```python
from build123d import *

# Parameters (mm, degrees)
BOSS_EXTRUDE1_DEPTH = 146.05
BOSS_EXTRUDE2_DEPTH = 6.35
SKETCH3_W           = 274.391313821
SKETCH3_H           = 212.158232336
CUT_EXTRUDE1_DEPTH  = 81.28
SKETCH4_W           = 56.814403599
SKETCH4_H           = 146.05
SKETCH4_W_2         = 112.041307198
CUT_EXTRUDE2_DEPTH  = 269.802733384


with BuildPart() as part:
    # Sketch1 → Boss-Extrude1 (new body)
    with BuildSketch(Plane.XY):
        Polygon((0, 0), (0, 107.95), (3.175, 107.95), (7.6109518, 6.35), (50.7909518, 6.35), (55.226903599, 107.95), (58.401903599, 107.95), (62.837855399, 6.35), (106.017855399, 6.35), (110.453807198, 107.95), (113.628807198, 107.95), (118.064758998, 6.35), (161.244758998, 6.35), (165.680710797, 107.95), (168.855710797, 107.95), (173.291662597, 6.35), (216.471662597, 6.35), (220.907614396, 107.95), (224.082614396, 107.95), (224.082614396, 0), align=None)
    extrude(amount=BOSS_EXTRUDE1_DEPTH)

    # Sketch2 → Boss-Extrude2 (add)
    with BuildSketch(Plane.XY.offset(146.05)):
        Polygon((3.175, 107.95), (55.226903599, 107.95), (50.7909518, 6.35), (7.6109518, 6.35), align=None)
        Polygon((58.401903599, 107.95), (62.837855399, 6.35), (106.017855399, 6.35), (110.453807198, 107.95), align=None)
        Polygon((113.628807198, 107.95), (118.064758998, 6.35), (161.244758998, 6.35), (165.680710797, 107.95), align=None)
        Polygon((168.855710797, 107.95), (173.291662597, 6.35), (216.471662597, 6.35), (220.907614396, 107.95), align=None)
    boss_extrude2 = extrude(amount=-BOSS_EXTRUDE2_DEPTH)

    # Mirror1: Boss-Extrude2 across plane
    add(boss_extrude2.mirror(Plane(origin=(0, 0, 73.025), x_dir=(1, 0, 0), z_dir=(0, 0, -1))))

    # Sketch3 → Cut-Extrude1 (cut)
    with BuildSketch(Plane(origin=(0, 107.95, 0), x_dir=(1, 0, 0), z_dir=(0, 1, 0))):
        with Locations((112.984880501, -67.937773638)):
            Rectangle(SKETCH3_W, SKETCH3_H)
    extrude(amount=-CUT_EXTRUDE1_DEPTH, mode=Mode.SUBTRACT)

    # Sketch4 → Cut-Extrude2 (cut, through all)
    with BuildSketch(Plane(origin=(0, 26.67, 0), x_dir=(1, 0, 0), z_dir=(0, 1, 0))):
        with Locations((28.4072018, -73.025)):
            Rectangle(SKETCH4_W, SKETCH4_H)
        with Locations((168.061960797, -73.025)):
            Rectangle(SKETCH4_W_2, SKETCH4_H)
    extrude(amount=-CUT_EXTRUDE2_DEPTH, mode=Mode.SUBTRACT)


solid = part.part
```
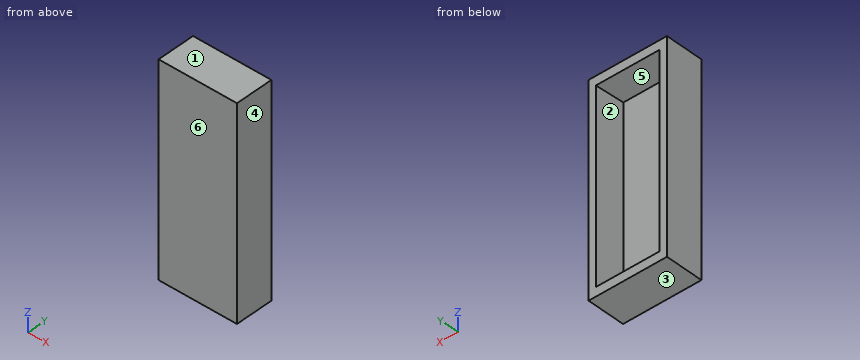
The model under review builds one solid part; all positions refer to its coordinate system, in mm. Face numbers are marked on the shaded views. A direction names the side the tool comes from. Give positions to 0.01 mm unless a question says otherwise; leave off trailing zeros. Write each loop counter-clockwise with the first axis right and the second up, starting at its lowest first coordinate (ties: lowest second). Pieces come first, ordered by that corner, then holes. Notation, with made-up numbers: (52, -10.75) -> (86, -10.75) arc R20 ccw to (86, 20.25) -> close; hole circle Ø10 at (4.25, 0.25). An arc over 180 degrees is marked (long way). Answer in a Markdown table with one row per item.
1) For L1, parallel to Z at x = 72, y = 23.25; L2, parallel to Y at x = 103.5, z = 92.5; L3, parallel to X at y = 15, z = 133, list the stretches that pass through material, from the lowest coordinate up. Write a range as [from, to].
Worked answers:
| item | result |
|---|---|
| L1 | [0, 6.35], [139.7, 146.05] |
| L2 | [0, 6.35] |
| L3 | [56.81, 62.46], [106.4, 112.04] |
2) Add section C-C on x = 85. State the section outline as (y, z) points.
Worked answers:
| item | result |
|---|---|
| outline | (0, 0) -> (26.67, 0) -> (26.67, 6.35) -> (6.35, 6.35) -> (6.35, 139.7) -> (26.67, 139.7) -> (26.67, 146.05) -> (0, 146.05) -> close |
3) Clearance check with a flat-ended pin moving along its axis: P1, Ø2, axis at x = 92.5, z = 22.5, coming from the +Y side. State where the tip first meets the part, or that it passes through.
Worked answers:
| item | result |
|---|---|
| P1 | y = 6.35 |
4) Tool access review of the marked faces 5 and 6: name each direction out of +Z, -Z, +X, -X, +Y, -Y from which nothing blocks a thin tool from reaching the whole face with its end or side.
Worked answers:
| item | result |
|---|---|
| face 5 | +Y |
| face 6 | +Z, -Z, +X, -X, -Y |
5) Add section B-B on z = 137.5. State the section outline as (x, y) points, plus the area to 3 significant figures.
Worked answers:
| item | result |
|---|---|
| outline | (56.81, 0) -> (112.04, 0) -> (112.04, 26.67) -> (106.91, 26.67) -> (106.02, 6.35) -> (62.84, 6.35) -> (61.95, 26.67) -> (56.81, 26.67) -> close |
| area | 577 mm² |
6) Mouldability with a two-part tool opening along Z and no side actions: class the marked faces 1, 2, 3 and 4 as +Z half, -Z half, draft (parallel to the pull), parting line (faces both ways), or undercut.
Worked answers:
| item | result |
|---|---|
| face 1 | +Z half |
| face 2 | undercut |
| face 3 | -Z half |
| face 4 | draft |
7) Add section A-A on y = 25. State the section outline as (x, z) points, plus the area to 3 significant figures.
Worked answers:
| item | result |
|---|---|
| outline | (56.81, 0) -> (112.04, 0) -> (112.04, 146.05) -> (56.81, 146.05) -> close; hole (62.02, 6.35) -> (106.83, 6.35) -> (106.83, 139.7) -> (62.02, 139.7) -> close |
| area | 2,090 mm² |
8) Add section D-D on y = 14.75. State the section outline as (x, z) points, plus the area to 3 significant figures.
Worked answers:
| item | result |
|---|---|
| outline | (56.81, 0) -> (112.04, 0) -> (112.04, 146.05) -> (56.81, 146.05) -> close; hole (62.47, 6.35) -> (106.38, 6.35) -> (106.38, 139.7) -> (62.47, 139.7) -> close |
| area | 2,210 mm² |
